Build history of the part. All positions in model axes, mm. Give positions to 0.01 mm unless a question says otherwise; leave off trailing zeros. Order: outer loops, then holes, each group sorted by start corner. A loop starts at its lowest first (then second) coordinate and runs counter-clockwise, first axis right, second up. Notation, with made-up numbers: (74, -29.5) - (128, -29.5) arc R26 ccw to (128, -10.5) - close; hole circle Ø5 at (43.5, 31). An arc over 180 degrees is marked (long way). Use a Markdown table: item, result. Add a question column.
(1) Mould opens along X. For faces 1 (the face through (-41.265, -31.641, -99.014)), 2 (the face through (-0.7, 12.3, -100)), 3 (the face through (-40.097, -16.961, -99.014)) say: +X half, -X half, draft (parallel to the pull), parting line (faces both ways), or undercut.
(2) Wall check: line 1 (Y direction, x = 0, z = -99.1); line 2 (X direction, y = -16, z = -99.3); line 3 (X direction, y = -0.5, z = -99.7). Give the ranges that are in metal, low to high.
(3) Flat gauge pins, fed straight in: pin 1 (1 mm diameter, centred on x = 26, z = -99.5, fed in from -Y); pin 2 (1.8 mm diameter, centred on x = 0, y = -16, fed in from -Z) (3 decimals). Where does each tip first touch, or does it go through?
(4) Slice it at B-B (y = -3). Write the cut outline in (x, z), then the cut area to 3 significant figures.
(5) Slice it at A-A (x = -5.5). Write the cut outline in (y, z).
(6) Slice it at C-C (z = -98.4). Count the separate pieces of the cut face and the enclosed holes in it, then the cut area to 3 significant figures.
(7) Slice it at D-D (y = 31.5). Write the cut outline in (x, z), then the cut area to 3 significant figures.
from build123d import *

# Parameters (mm, degrees)
CYLINDER623_R               = 1.5
CYLINDER623_DEPTH           = 20
CYLINDER623_PLACEMENT_ANGLE = 45
CYLINDER632_R               = 1.5
CYLINDER632_DEPTH           = 20
CYLINDER629_R               = 1.5
CYLINDER629_DEPTH           = 20
CYLINDER629_PLACEMENT_ANGLE = 135
CYLINDER639_R               = 1.5
CYLINDER639_DEPTH           = 20
CYLINDER638_R               = 1.5
CYLINDER638_DEPTH           = 20
CYLINDER638_PLACEMENT_ANGLE = 225
CYLINDER631_R               = 1.5
CYLINDER631_DEPTH           = 20
CYLINDER633_R               = 1.5
CYLINDER633_DEPTH           = 20
CYLINDER633_PLACEMENT_ANGLE = 45
CYLINDER628_R               = 1.5
CYLINDER628_DEPTH           = 20
COMPOUND654_PLACEMENT_ANGLE = 22.5
CYLINDER625_R               = 1.5
CYLINDER625_DEPTH           = 16
CYLINDER625_PLACEMENT_ANGLE = 67.5
CYLINDER626_R               = 1.5
CYLINDER626_DEPTH           = 16
CYLINDER626_PLACEMENT_ANGLE = 22.5
CYLINDER627_R               = 1.5
CYLINDER627_DEPTH           = 16
CYLINDER627_PLACEMENT_ANGLE = 112.5
CYLINDER630_R               = 1.5
CYLINDER630_DEPTH           = 16
CYLINDER630_PLACEMENT_ANGLE = 202.5
TUBE038_R                   = 52
TUBE038_R_2                 = 12
TUBE038_DEPTH               = 2


with BuildPart() as obj1:
    # Cylinder623 → Cylinder623 (new body)
    with BuildSketch(Plane.XY):
        Circle(CYLINDER623_R)
    extrude(amount=CYLINDER623_DEPTH)


with BuildPart() as obj1_1:
    # Cylinder623 placement: moved
    add(obj1.part.moved(Location((-31.819805, 31.819805, -18))).rotate(Axis((-31.819805, 31.819805, -18), (0, 0, 1)), CYLINDER623_PLACEMENT_ANGLE))


with BuildPart() as obj2:
    # Cylinder632 → Cylinder632 (new body)
    with BuildSketch(Plane(origin=(-45, 0, -18), x_dir=(0, 1, 0), z_dir=(0, 0, 1))):
        Circle(CYLINDER632_R)
    extrude(amount=CYLINDER632_DEPTH)


with BuildPart() as obj3:
    # Cylinder629 → Cylinder629 (new body)
    with BuildSketch(Plane.XY):
        Circle(CYLINDER629_R)
    extrude(amount=CYLINDER629_DEPTH)


with BuildPart() as obj3_1:
    # Cylinder629 placement: moved
    add(obj3.part.moved(Location((-31.819805, -31.819805, -18))).rotate(Axis((-31.819805, -31.819805, -18), (0, 0, 1)), CYLINDER629_PLACEMENT_ANGLE))


with BuildPart() as obj4:
    # Cylinder639 → Cylinder639 (new body)
    with BuildSketch(Plane(origin=(0, -45, -18), x_dir=(-1, 0, 0), z_dir=(0, 0, 1))):
        Circle(CYLINDER639_R)
    extrude(amount=CYLINDER639_DEPTH)


with BuildPart() as obj5:
    # Cylinder638 → Cylinder638 (new body)
    with BuildSketch(Plane.XY):
        Circle(CYLINDER638_R)
    extrude(amount=CYLINDER638_DEPTH)


with BuildPart() as obj5_1:
    # Cylinder638 placement: moved
    add(obj5.part.moved(Location((31.819805, -31.819805, -18))).rotate(Axis((31.819805, -31.819805, -18), (0, 0, 1)), CYLINDER638_PLACEMENT_ANGLE))


with BuildPart() as obj6:
    # Cylinder631 → Cylinder631 (new body)
    with BuildSketch(Plane(origin=(45, 0, -18), x_dir=(0, -1, 0), z_dir=(0, 0, 1))):
        Circle(CYLINDER631_R)
    extrude(amount=CYLINDER631_DEPTH)


with BuildPart() as obj7:
    # Cylinder633 → Cylinder633 (new body)
    with BuildSketch(Plane.XY):
        Circle(CYLINDER633_R)
    extrude(amount=CYLINDER633_DEPTH)


with BuildPart() as obj7_1:
    # Cylinder633 placement: moved
    add(obj7.part.moved(Location((31.819805, 31.819805, -18))).rotate(Axis((31.819805, 31.819805, -18), (0, 0, -1)), CYLINDER633_PLACEMENT_ANGLE))


with BuildPart() as compound654:
    # Cylinder628 → Cylinder628 (new body)
    with BuildSketch(Plane(origin=(0, 45, -18), x_dir=(1, 0, 0), z_dir=(0, 0, 1))):
        Circle(CYLINDER628_R)
    extrude(amount=CYLINDER628_DEPTH)

    # Compound654: union obj1, obj2, obj3, obj4, obj5, obj6, obj7
    add(obj1_1.part)
    add(obj2.part)
    add(obj3_1.part)
    add(obj4.part)
    add(obj5_1.part)
    add(obj6.part)
    add(obj7_1.part)


with BuildPart() as compound654_1:
    # Compound654 placement: moved
    add(compound654.part.moved(Location((0, 0, -87))).rotate(Axis((0, 0, -87), (0, 0, 1)), COMPOUND654_PLACEMENT_ANGLE))


with BuildPart() as obj8:
    # Cylinder625 → Cylinder625 (new body)
    with BuildSketch(Plane.XY):
        Circle(CYLINDER625_R)
    extrude(amount=CYLINDER625_DEPTH)


with BuildPart() as obj8_1:
    # Cylinder625 placement: moved
    add(obj8.part.moved(Location((0, 16, 2))).rotate(Axis((0, 16, 2), (0, 0, -1)), CYLINDER625_PLACEMENT_ANGLE))


with BuildPart() as obj9:
    # Cylinder626 → Cylinder626 (new body)
    with BuildSketch(Plane.XY):
        Circle(CYLINDER626_R)
    extrude(amount=CYLINDER626_DEPTH)


with BuildPart() as obj9_1:
    # Cylinder626 placement: moved
    add(obj9.part.moved(Location((-16, 0, 2))).rotate(Axis((-16, 0, 2), (0, 0, 1)), CYLINDER626_PLACEMENT_ANGLE))


with BuildPart() as obj10:
    # Cylinder627 → Cylinder627 (new body)
    with BuildSketch(Plane.XY):
        Circle(CYLINDER627_R)
    extrude(amount=CYLINDER627_DEPTH)


with BuildPart() as obj10_1:
    # Cylinder627 placement: moved
    add(obj10.part.moved(Location((0, -16, 2))).rotate(Axis((0, -16, 2), (0, 0, 1)), CYLINDER627_PLACEMENT_ANGLE))


with BuildPart() as compound653:
    # Cylinder630 → Cylinder630 (new body)
    with BuildSketch(Plane.XY):
        Circle(CYLINDER630_R)
    extrude(amount=CYLINDER630_DEPTH)


with BuildPart() as compound653_1:
    # Cylinder630 placement: moved
    add(compound653.part.moved(Location((16, 0, 2))).rotate(Axis((16, 0, 2), (0, 0, 1)), CYLINDER630_PLACEMENT_ANGLE))

    # Compound653: union obj8, obj9, obj10
    add(obj8_1.part)
    add(obj9_1.part)
    add(obj10_1.part)


with BuildPart() as compound653_2:
    # Compound653 placement: moved
    add(compound653_1.part.moved(Location((0, 0, -111))))


with BuildPart() as cut287:
    # Tube038 → Tube038 (new body)
    with BuildSketch(Plane.XY.offset(-100)):
        Circle(TUBE038_R)
        Circle(TUBE038_R_2, mode=Mode.SUBTRACT)
    extrude(amount=TUBE038_DEPTH)

    # Cut285: cut Compound653
    add(compound653_2.part, mode=Mode.SUBTRACT)

    # Cut287: cut Compound654
    add(compound654_1.part, mode=Mode.SUBTRACT)


solid = cut287.part
Solution:
| question | item | result |
|---|---|---|
| 1 | face 1 | parting line |
| 1 | face 2 | draft |
| 1 | face 3 | undercut |
| 2 | line 1 | -52 to -17.5, -14.5 to -12, 12 to 14.5, 17.5 to 52 |
| 2 | line 2 | -49.48 to -42.45, -40.7 to -1.5, 1.5 to 40.7, 42.45 to 49.48 |
| 2 | line 3 | -52 to -17.41, -14.59 to -11.99, 11.99 to 14.59, 17.41 to 52 |
| 3 | pin 1 | y = -45.32 |
| 3 | pin 2 | through |
| 4 | outline | (-51.91, -100) - (-11.62, -100) - (-11.62, -98) - (-51.91, -98) - close; (11.62, -100) - (51.91, -100) - (51.91, -98) - (11.62, -98) - close |
| 4 | area | 161 mm2 |
| 5 | outline | (-51.71, -100) - (-10.67, -100) - (-10.67, -98) - (-51.71, -98) - close; (10.67, -100) - (51.71, -100) - (51.71, -98) - (10.67, -98) - close |
| 6 | separate pieces | 1 |
| 6 | enclosed holes | 13 |
| 6 | area | 7,960 mm2 |
| 7 | outline | (-41.37, -100) - (41.37, -100) - (41.37, -98) - (-41.37, -98) - close |
| 7 | area | 165 mm2 |
